Can you work these out from the model? Positions are in its coordinate system, mm. A direction names the side the tool comes from. Round coordinates to 2 decimals unless told otherwise and drop trailing zeros. Loops run counter-clockwise (first coordinate to the right, second up) from the corner with the lowest first, then second, coordinate; pieces in that order, holes last.
(1) If I drill on line 1 along X through (y, z) = (-22.5, 2.8) (3 decimals); line 2 along Y through (x, z) = (-21, -0.6); line 3 along X through (y, z) = (-2, -0.4) (3 decimals), over which ranges is the centre line in solid material (lowest first)?
(2) Thinking about a two-plate mould opening in Y: for faces 1 (the face through (-73.39, -32.05, 0.79)), 2 (the face through (76.843, 42.095, -1.014)), 3 (the face through (74.245, 5, 1)), 4 (the face through (0, -38, 0)), which applies, released by +Y, released by -Y, zero draft, split by the parting line, or undercut?
(3) Will these pins go through, and if not, where does the flat tip stop? pin 1 Ø1.6 at (y, z) = (3.5, -0.5) entering from +X (3 decimals); pin 2 Ø0.6 at (x, z) = (2.5, -0.5) entering from -Y; pin 3 Ø0.6 at (y, z) = (-0.5, -0.5) entering from -X (3 decimals); pin 4 Ø1.6 at (y, z) = (-12, -1) entering from +X (3 decimals).
(4) I want a section at C-C on x = 65. Write out the boundary of the cut face in (y, z), plus the area to 4 significant figures.
(5) I want a section at B-B on z = 2.45. Write out the boundary of the cut face in (x, y) (3 decimals), plus the area to 3 significant figures.
(6) Which directions (+Z, -Z, +X, -X, +Y, -Y) give clear straight access to the entire face, cutting with the end or side of a thin tool? Please do faces 5 (the face through (-76.843, 42.095, -1.014)), 6 (the face through (-83.39, 38.55, 2.51)), 7 (the face through (1, 41, 0)), 8 (the face through (73.39, 38.55, -1.01)).
(7) I want a section at A-A on y = 13.5. Write out the boundary of the cut face in (x, z) (3 decimals), plus the area to 3 significant figures.
from build123d import *

# Parameters (mm, degrees)
SKETCH1_W           = 168.49
SKETCH1_H           = 85.9
BOSS_EXTRUDE1_DEPTH = 3.5
SKETCH2_W           = 148.49
SKETCH2_H           = 75.9
CUT_EXTRUDE1_DEPTH  = 3.5
SKETCH4_W           = 3.5
SKETCH4_H           = 1.5
BOSS_EXTRUDE2_DEPTH = 148.49
SKETCH5_W           = 2
SKETCH5_H           = 2
CUT_EXTRUDE2_DEPTH  = 176.5
FILLET3_R           = 3
FILLET4_R           = 3
SKETCH6_W           = 155.49
SKETCH6_H           = 79.4
SKETCH6_W_2         = 148.49
SKETCH6_H_2         = 72.4
BOSS_EXTRUDE3_DEPTH = 2
FILLET5_R           = 3
FILLET6_R           = 3
FILLET7_R           = 3
FILLET8_R           = 3


with BuildPart() as part:
    # Sketch1 → Boss-Extrude1 (new body)
    with BuildSketch(Plane.XY):
        Rectangle(SKETCH1_W, SKETCH1_H)
    extrude(amount=BOSS_EXTRUDE1_DEPTH)

    # Sketch2 → Cut-Extrude1 (cut)
    with BuildSketch(Plane.XY.offset(3.5)):
        with Locations((0, 5)):
            Rectangle(SKETCH2_W, SKETCH2_H)
    extrude(amount=-CUT_EXTRUDE1_DEPTH, mode=Mode.SUBTRACT)

    # Sketch4 → Boss-Extrude2 (add)
    with BuildSketch(Plane.ZY.offset(-74.245)):
        with Locations((1.75, 42.2)):
            Rectangle(SKETCH4_W, SKETCH4_H)
    extrude(amount=BOSS_EXTRUDE2_DEPTH)

    # Sketch5 → Cut-Extrude2 (cut)
    with BuildSketch(Plane(origin=(84.245, 0, 0), x_dir=(0, 0, -1), z_dir=(1, 0, 0))):
        with Locations((-2.5, 40.45)):
            Rectangle(SKETCH5_W, SKETCH5_H)
    extrude(amount=-CUT_EXTRUDE2_DEPTH, mode=Mode.SUBTRACT)

    # Fillet3
    fillet3_edges = [part.edges().sort_by_distance(p)[0] for p in [
        (-84.245, -42.95, 1.75),
    ]]
    fillet(fillet3_edges, radius=FILLET3_R)

    # Fillet4
    fillet4_edges = [part.edges().sort_by_distance(p)[0] for p in [
        (-84.245, 39.45, 2.5),
        (84.245, -42.95, 1.75),
    ]]
    fillet(fillet4_edges, radius=FILLET4_R)

    # Sketch6 → Boss-Extrude3 (add)
    with BuildSketch(Plane(origin=(0, 0, 0), x_dir=(-1, 0, 0), z_dir=(0, 0, -1))):
        with Locations((0, 3.25)):
            Rectangle(SKETCH6_W, SKETCH6_H)
        with Locations((0, 3.25)):
            Rectangle(SKETCH6_W_2, SKETCH6_H_2, mode=Mode.SUBTRACT)
    extrude(amount=BOSS_EXTRUDE3_DEPTH)

    # Fillet5
    fillet5_edges = [part.edges().sort_by_distance(p)[0] for p in [
        (84.245, 39.45, 2.5),
    ]]
    fillet(fillet5_edges, radius=FILLET5_R)

    # Fillet6
    fillet6_edges = [part.edges().sort_by_distance(p)[0] for p in [
        (-84.245, 42.95, 1.75),
        (84.245, 42.95, 1.75),
    ]]
    fillet(fillet6_edges, radius=FILLET6_R)

    # Fillet7
    fillet7_edges = [part.edges().sort_by_distance(p)[0] for p in [
        (77.745, 42.95, -1),
        (77.745, -36.45, -1),
        (-77.745, -36.45, -1),
        (-77.745, 42.95, -1),
    ]]
    fillet(fillet7_edges, radius=FILLET7_R)

    # Fillet8
    fillet8_edges = [part.edges().sort_by_distance(p)[0] for p in [
        (74.245, 39.45, -1),
        (-74.245, 39.45, -1),
        (-74.245, -32.95, 0.75),
        (74.245, -32.95, 0.75),
    ]]
    fillet(fillet8_edges, radius=FILLET8_R)


solid = part.part
Filled sheet:
1. line 1: x = -84.245 to -74.245, 74.245 to 84.245
1. line 2: y = -36.45 to -32.95, 39.45 to 42.95
1. line 3: x = -77.745 to -74.245, 74.245 to 77.745
2. face 1: undercut
2. face 2: released by +Y
2. face 3: undercut
2. face 4: zero draft
3. pin 1: stops at x = 84.245
3. pin 2: stops at y = -36.45
3. pin 3: stops at x = -77.745
3. pin 4: stops at x = 77.745
4. outline: (-42.95, 0) - (-36.45, 0) - (-36.45, -2) - (-32.95, -2) - (-32.95, 3.5) - (-42.95, 3.5) - close; (39.45, -2) - (42.95, -2) - (42.95, 3.5) - (41.45, 3.5) - (41.45, 0) - (39.45, 0) - close
4. area: 54.25 mm2
5. outline: (-84.245, -39.95) arc R3 ccw to (-81.245, -42.95) - (81.245, -42.95) arc R3 ccw to (84.245, -39.95) - (84.245, 36.45) arc R3 ccw to (81.245, 39.45) - (74.245, 39.45) - (74.245, -29.95) arc R3 cw to (71.245, -32.95) - (-71.245, -32.95) arc R3 cw to (-74.245, -29.95) - (-74.245, 39.45) - (-81.245, 39.45) arc R3 ccw to (-84.245, 36.45) - close; (-83.843, 41.45) - (83.843, 41.45) arc R3 ccw to (81.245, 42.95) - (-81.245, 42.95) arc R3 ccw to start
5. area: 3,380 mm2
6. face 5: -Z, -X, +Y
6. face 6: +Z, -X
6. face 7: +Z
6. face 8: +Z, -Z
7. outline: (-84.245, 0) - (-77.745, 0) - (-77.745, -2) - (-74.245, -2) - (-74.245, 3.5) - (-84.245, 3.5) - close; (74.245, -2) - (77.745, -2) - (77.745, 0) - (84.245, 0) - (84.245, 3.5) - (74.245, 3.5) - close
7. area: 84.0 mm2
